Verification items for the finished model (mm, model axes). Give positions to 0.01 mm unless a question says otherwise; leave off trailing zeros. Write each loop counter-clockwise with the first axis right and the second up, starting at its lowest first coordinate (ties: lowest second). Pieces come first, ordered by that corner, then holes. Notation, with made-up numbers: (48.25, 24.5) -> (105.25, 24.5) arc R14 ccw to (105.25, 43.5) -> close; hole circle Ø10 at (82.5, 32). An arc over 180 degrees is marked (long way). Answer as CSV lines item,"result".
```python
from build123d import *

# Parameters (mm, degrees)
SKETCH1_R                            = 4.7625
BOSS_EXTRUDE1_DEPTH                  = 13.02131
F_10_32_TAPPED_HOLE2_D               = 4.0386
F_10_32_TAPPED_HOLE2_DEPTH           = 15.07744
F_10_32_TAPPED_HOLE2_TIP             = 1.213317848
F_10_32_TAPPED_HOLE2_ON_FACE_2_D     = 4.0386
F_10_32_TAPPED_HOLE2_ON_FACE_2_DEPTH = 15.07744
F_10_32_TAPPED_HOLE2_ON_FACE_2_TIP   = 1.213317848


with BuildPart() as part:
    # Sketch1 → Boss-Extrude1 (new, symmetric)
    with BuildSketch(Plane.XY):
        with Locations(Location((0, 0, 0), (0, 0, 180))):
            Circle(SKETCH1_R)
    extrude(amount=BOSS_EXTRUDE1_DEPTH, both=True)

    # #10-32 Tapped Hole2
    with Locations(Plane.XY.offset(13.02131)):
        with Locations((0, 0)):
            Hole(F_10_32_TAPPED_HOLE2_D / 2, depth=F_10_32_TAPPED_HOLE2_DEPTH)
            with Locations((0, 0, -(F_10_32_TAPPED_HOLE2_DEPTH + F_10_32_TAPPED_HOLE2_TIP / 2))):  # 118° drill point
                Cone(0, F_10_32_TAPPED_HOLE2_D / 2, F_10_32_TAPPED_HOLE2_TIP, mode=Mode.SUBTRACT)

    # #10-32 Tapped Hole2 on face 2
    with Locations(Plane(origin=(0, 0, -13.02131), x_dir=(-1, 0, 0), z_dir=(0, 0, -1))):
        with Locations((0, 0)):
            Hole(F_10_32_TAPPED_HOLE2_ON_FACE_2_D / 2, depth=F_10_32_TAPPED_HOLE2_ON_FACE_2_DEPTH)
            with Locations((0, 0, -(F_10_32_TAPPED_HOLE2_ON_FACE_2_DEPTH + F_10_32_TAPPED_HOLE2_ON_FACE_2_TIP / 2))):  # 118° drill point
                Cone(0, F_10_32_TAPPED_HOLE2_ON_FACE_2_D / 2, F_10_32_TAPPED_HOLE2_ON_FACE_2_TIP, mode=Mode.SUBTRACT)


solid = part.part
```
1) Depth check by flat-ended pin: pin 1 (3 mm diameter, centred on y = -1, z = -10, fed in from +X); pin 2 (1.5 mm diameter, centred on x = 1.5, z = 10.5, fed in from -Y); pin 3 (2 mm diameter, centred on y = -3, z = 5.5, fed in from -X); pin 4 (1.5 mm diameter, centred on x = -1, y = 0.5, fed in from -Z). Enter the tip coordinate at first touch or a pass-through.
Reported:
pin 1,"x = 4.76"
pin 2,"y = -4.7"
pin 3,"x = -4.32"
pin 4,"through"
2) Section check D-D (y = 4.25). Record the boundary of the cut face in (x, z), and give its area (3 significant figures).
Reported:
outline,"(-2.15, -13.02) -> (2.15, -13.02) -> (2.15, 13.02) -> (-2.15, 13.02) -> close"
area,"112 mm²"
3) Section check A-A (x = 0). Record the boundary of the cut face in (y, z).
Reported:
outline,"(-4.76, -13.02) -> (-2.02, -13.02) -> (-2.02, 13.02) -> (-4.76, 13.02) -> close; (2.02, -13.02) -> (4.76, -13.02) -> (4.76, 13.02) -> (2.02, 13.02) -> close"
4) Section check B-B (y = -1). Record the boundary of the cut face in (x, z).
Reported:
outline,"(-4.66, -13.02) -> (-1.75, -13.02) -> (-1.75, 13.02) -> (-4.66, 13.02) -> close; (1.75, -13.02) -> (4.66, -13.02) -> (4.66, 13.02) -> (1.75, 13.02) -> close"
5) Section check C-C (z = 4.5). Record the boundary of the cut face in (x, y) (1 decimal).
Reported:
outline,"circle Ø9.5 at (0, 0); hole circle Ø4 at (0, 0)"
6) Scan lines: line 1 along Y through (x, z) = (0, 7.5); line 2 along Y through (x, z) = (-0.5, 3); line 3 along X through (y, z) = (-0.75, 10.25). Record each from-to range of solid material in increasing order.
Reported:
line 1,"-4.76 to -2.02, 2.02 to 4.76"
line 2,"-4.74 to -1.96, 1.96 to 4.74"
line 3,"-4.7 to -1.87, 1.87 to 4.7"
